Input: part model. Units: mm. Frame: model coordinates. Face numbers are marked on the shaded views. A direction names the side the tool comes from. Give positions to 0.01 mm unless a question says otherwise; leave off trailing zeros. Write each loop counter-clockwise with the first axis right and the second up, starting at its lowest first coordinate (ties: lowest second). Pieces come first, ordered by that corner, then holes. Notation, with made-up numbers: (63.5, 13) - (81.5, 13) arc R14 cw to (81.5, 17) - close; hole circle Ø5 at (-10, 59). An arc over 180 degrees is marked (long way). Use a Markdown table: item, result. Add a question column.
1. Section query A-A, the plane y = -270. Return loops of the section in (x, z), plus the area to 3 significant figures.
2. Mould query, pull axis Z, two halves, no side actions, for the marked faces 5, 6 and 7. Classes: released by +Z, released by -Z, zero draft, split by the parting line, or undercut.
3. Pin query (flat end, axial travel): pin 1 (8 mm diameter, centred on x = -166, y = -42, fed in from -Z); pin 2 (2 mm diameter, centred on y = -84, z = 343.5, fed in from -X); pin 3 (10 mm diameter, centred on x = 15, z = 476.5, fed in from +Y); pin 4 (2.5 mm diameter, centred on y = 2, z = 39.5, fed in from -X). Return the tip coordinate at first contact, or that it passes through.
4. Section query D-D, the plane x = 29.5. Return loops of the section in (y, z), plus the area to 3 significant figures.
5. Set-up query: the marked faces 1, 2, 3 and 4. Return all of +Z, -Z, +X, -X, +Y, -Y with unobstructed straight access to the full face (end or side cutting, diameter ignored); none if empty.
6. Material intervals for probe 1 along Y at (x, z) = (270, 7); probe 2 along Z at (x, y) = (7, -70.5); probe 3 along X at (y, z) = (-157, 54.5), sorted ascending.
```python
from build123d import *

# Parameters (mm, degrees)
EXTRUDE004_DEPTH         = 30
SKETCH001_R              = 96.85
SKETCH001_R_2            = 86.85
EXTRUDE001_DEPTH         = 540
EXTRUDE002_DEPTH         = 4
ARRAY_COUNT              = 4
EXTRUDE003_DEPTH         = 4
ARRAY001_COUNT           = 4
ARRAY001_PLACEMENT_ANGLE = 45
SKETCH_W                 = 600
SKETCH_H                 = 600
SKETCH_R                 = 9
EXTRUDE_DEPTH            = 30


with BuildPart() as lastplatte:
    # Sketch004 (on Face51 of Fusion) → Extrude004 (new body)
    with BuildSketch(Plane.XY.offset(570)):
        Polygon((110, 63.50853), (0, 127.017059), (-110, 63.50853), (-110, -63.50853), (0, -127.017059), (110, -63.50853), align=None)
    extrude(amount=EXTRUDE004_DEPTH)


with BuildPart() as rohr:
    # Sketch001 (on Face10 of Extrude) → Extrude001 (new body)
    with BuildSketch(Plane.XY.offset(30)):
        Circle(SKETCH001_R)
        Circle(SKETCH001_R_2, mode=Mode.SUBTRACT)
    extrude(amount=EXTRUDE001_DEPTH)


with BuildPart() as obj1:
    # Sketch002 → Extrude002 (new body, symmetric)
    with BuildSketch(Plane.XZ):
        Polygon((114, 30), (94, 50), (94, 230), (159, 230), (279, 60), (279, 30), align=None)
    extrude(amount=EXTRUDE002_DEPTH, both=True)

    # Array: obj1 ×4 about axis
    array_axis = Axis((0, 0, 0), (0, 0, 1))


with BuildPart() as obj1_1:
    add(obj1.part)
    for i in range(1, ARRAY_COUNT):
        add(obj1.part.rotate(array_axis, i * 360 / ARRAY_COUNT))


with BuildPart() as obj2:
    # Sketch003 → Extrude003 (new body, symmetric)
    with BuildSketch(Plane.XZ):
        Polygon((114, 30), (94, 50), (94, 230), (159, 230), (344, 60), (344, 30), align=None)
    extrude(amount=EXTRUDE003_DEPTH, both=True)

    # Array001: obj2 ×4 about axis
    array001_axis = Axis((0, 0, 0), (0, 0, 1))


with BuildPart() as obj2_1:
    add(obj2.part)
    for i in range(1, ARRAY001_COUNT):
        add(obj2.part.rotate(array001_axis, i * 360 / ARRAY001_COUNT))


with BuildPart() as obj2_2:
    # Array001 placement: moved
    add(obj2_1.part.rotate(Axis((0, 0, 0), (0, 0, 1)), ARRAY001_PLACEMENT_ANGLE))


with BuildPart() as fusion001:
    # Sketch → Extrude (new body)
    with BuildSketch(Plane.XY):
        Rectangle(SKETCH_W, SKETCH_H)
        with Locations((270, -270)):
            Circle(SKETCH_R, mode=Mode.SUBTRACT)
        with Locations((-270, -270)):
            Circle(SKETCH_R, mode=Mode.SUBTRACT)
        with Locations((270, 270)):
            Circle(SKETCH_R, mode=Mode.SUBTRACT)
        with Locations((-270, 270)):
            Circle(SKETCH_R, mode=Mode.SUBTRACT)
    extrude(amount=EXTRUDE_DEPTH)

    # Fusion: union rohr, obj1, obj2
    add(rohr.part)
    add(obj1_1.part)
    add(obj2_2.part)

    # Fusion001: union lastplatte
    add(lastplatte.part)


solid = fusion001.part
```
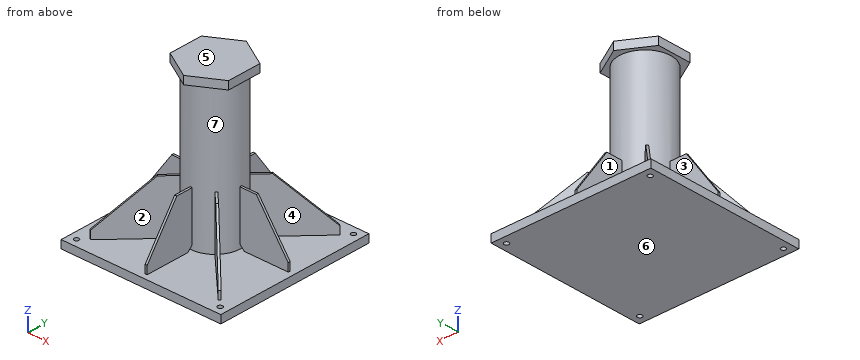
Result sheet:
| question | item | result |
|---|---|---|
| 1 | outline | (-300, 0) - (-279, 0) - (-279, 30) - (-300, 30) - close; (-261, 0) - (261, 0) - (261, 30) - (4, 30) - (4, 72.75) - (-4, 72.75) - (-4, 30) - (-261, 30) - close; (279, 0) - (300, 0) - (300, 30) - (279, 30) - close |
| 1 | area | 17,300 mm² |
| 2 | face 5 | released by +Z |
| 2 | face 6 | released by -Z |
| 2 | face 7 | undercut |
| 3 | pin 1 | stops at z = 0 |
| 3 | pin 2 | stops at x = -49.91 |
| 3 | pin 3 | stops at y = 96.33 |
| 3 | pin 4 | stops at x = -279 |
| 4 | outline | (-300, 0) - (300, 0) - (300, 30) - (92.25, 30) - (92.25, 570) - (109.99, 570) - (109.99, 600) - (-109.99, 600) - (-109.99, 570) - (-92.25, 570) - (-92.25, 30) - (-300, 30) - close; hole (-81.69, 30) - (81.69, 30) - (81.69, 570) - (-81.69, 570) - close |
| 4 | area | 36,000 mm² |
| 5 | face 1 | +Y |
| 5 | face 2 | -Y |
| 5 | face 3 | -X |
| 5 | face 4 | +X |
| 6 | probe 1 | y = -300 to -279, -261 to 261, 279 to 300 |
| 6 | probe 2 | z = 0 to 30, 570 to 600 |
| 6 | probe 3 | x = -162.66 to -151.34, -4 to 4, 151.34 to 162.66 |
